Could you check a few things on this model? Use its own coordinates, in mm. Give positions to 0.01 mm unless a question says otherwise; leave off trailing zeros. Order: outer loops, then holes, each group sorted by start corner. A loop starts at its lowest first (then second) coordinate and runs counter-clockwise, first axis right, second up.
(1) If we mould it in two halves opening along Y, with no side actions, what happens to faces 1 (the cylindrical face through (-27.715, 21.251, 0.783)), 2 (the cylindrical face through (26.763, -15.213, 0.805)), 3 (the flat face through (7, 0, 0))? For each: released by +Y, released by -Y, zero draft, split by the parting line, or undercut.
(2) If I drill on probe 1 along Y at (x, z) = (0, 0.4) (1 decimal); probe 2 along X at (y, z) = (-3, 0.5); probe 3 along X at (y, z) = (-1, 1.15), over which ranges is the centre line in solid material (lowest first)?
(3) Imagine slicing it at A-A, the plane y = 0. Write out the boundary of the cut face in (x, z) (1 decimal), then the cut area to 3 significant figures.
(4) Imagine slicing it at D-D, the plane y = -29.21. Write out the boundary of the cut face in (x, z), then the cut area to 3 significant figures.
(5) Imagine slicing it at C-C, the plane z = 1.3. State how many separate pieces and enclosed holes the cut face has, then the cut area to 3 significant figures.
(6) Imagine slicing it at B-B, the plane x = 0. Write out the boundary of the cut face in (y, z) (1 decimal), then the cut area to 3 significant figures.
Autodesk Inventor part; units mm, degrees
ref_plane "YZ Plane" through (0, 0, 0) normal (1, 0, 0) x (0, 1, 0)
ref_plane "XZ Plane" through (0, 0, 0) normal (0, 1, 0) x (-1, 0, 0)
ref_plane "XY Plane" through (0, 0, 0) normal (0, 0, 1) x (1, 0, 0)
sketch "Sketch1" plane through (0, 0, 0) normal (0, 0, 1) x (1, 0, 0)
  circle A0 centre (0, 0) radius 34.925
  dimension "d0" = 69.85
extrude "Extrusion1" add sketch "Sketch1" along normal blind 1.5875
sketch "Sketch2" plane through (0, 0, 1.5875) normal (0, 0, 1) x (1, 0, 0)
  line L0 (0, 0) -> (0, 29.21)
  circle A0 centre (0, 29.21) radius 1.5875
  circle A1 centre (-25.2966, 14.605) radius 1.5875
  circle A2 centre (-25.2966, -14.605) radius 1.5875
  circle A3 centre (0, -29.21) radius 1.5875
  circle A4 centre (25.2966, -14.605) radius 1.5875
  circle A5 centre (25.2966, 14.605) radius 1.5875
  dimension "d3" = 29.21
  dimension "d4" = 3.175
  dimension "d7" = 360
extrude "Extrusion2" cut sketch "Sketch2" against normal blind 2.4765
sketch "Sketch3" plane through (0, 0, 0) normal (0, 0, -1) x (-1, 0, 0)
  line L0 (0, 0) -> (25.4, 0)
  circle A0 centre (25.4, 0) radius 5.715
  dimension "d11" = 25.4
  dimension "d12" = 11.43
extrude "Extrusion3" cut sketch "Sketch3" against normal blind 2.4765
sketch "Sketch4" plane through (0, 0, 0) normal (0, 0, -1) x (-1, 0, 0)
  circle A0 centre (0, 0) radius 3.9624
  dimension "d15" = 7.9248
extrude "Extrusion4" cut sketch "Sketch4" against normal blind 2.4765
properties part number "pistonSealingWallFront" material "ABS Plastic"
Answer block:
1. face 1: split by the parting line
1. face 2: undercut
1. face 3: zero draft
2. probe 1: y = -34.9 to -30.8, -27.6 to -4, 4 to 27.6, 30.8 to 34.9
2. probe 2: x = -34.8 to -30.26, -20.54 to -2.59, 2.59 to 34.8
2. probe 3: x = -34.91 to -31.03, -19.77 to -3.83, 3.83 to 34.91
3. outline: (-34.9, 0) - (-31.1, 0) - (-31.1, 1.6) - (-34.9, 1.6) - close; (-19.7, 0) - (-4, 0) - (-4, 1.6) - (-19.7, 1.6) - close; (4, 0) - (34.9, 0) - (34.9, 1.6) - (4, 1.6) - close
3. area: 80.2 mm2
4. outline: (-19.15, 0) - (-1.59, 0) - (-1.59, 1.59) - (-19.15, 1.59) - close; (1.59, 0) - (19.15, 0) - (19.15, 1.59) - (1.59, 1.59) - close
4. area: 55.7 mm2
5. separate pieces: 1
5. enclosed holes: 8
5. area: 3,630 mm2
6. outline: (-34.9, 0) - (-30.8, 0) - (-30.8, 1.6) - (-34.9, 1.6) - close; (-27.6, 0) - (-4, 0) - (-4, 1.6) - (-27.6, 1.6) - close; (4, 0) - (27.6, 0) - (27.6, 1.6) - (4, 1.6) - close; (30.8, 0) - (34.9, 0) - (34.9, 1.6) - (30.8, 1.6) - close
6. area: 88.2 mm2
